```python
from build123d import *

# Parameters (mm, degrees)
BOSS_EXTRUDE1_DEPTH = 10
SKETCH1_5_OUTSIDE_W = 85.55
SKETCH1_5_OUTSIDE_H = 68.8
CUT_EXTRUDE2_DEPTH  = 10
SKETCH5_R           = 2.25
CUT_EXTRUDE3_DEPTH  = 10


with BuildPart() as part:
    # Sketch1 → Boss-Extrude1 (new body)
    with BuildSketch(Plane(origin=(0, 0, 0), x_dir=(0, 0, -1), z_dir=(1, 0, 0))):
        with BuildLine():
            Line((7.980196803, 33.697050156), (-4.769859567, -10.767680589))
            ThreePointArc((-4.769859567, -10.767680589), (-4.949582903, -11.029179666), (-5.250490415, -11.129861911))
            Line((-5.250490415, -11.129861911), (-12.87371339, -11.129861911))
            ThreePointArc((-12.87371339, -11.129861911), (-13.227266781, -11.276308521), (-13.37371339, -11.629861911))
            Line((-13.37371339, -11.629861911), (-13.37371339, -14.129861911))
            Line((-13.37371339, -14.129861911), (25.12628661, -14.129861911))
            Line((25.12628661, -14.129861911), (25.12628661, -11.629861911))
            ThreePointArc((25.12628661, -11.629861911), (24.979840001, -11.276308521), (24.62628661, -11.129861911))
            Line((24.62628661, -11.129861911), (17.12628661, -11.129861911))
            ThreePointArc((17.12628661, -11.129861911), (16.772733219, -10.983415302), (16.62628661, -10.629861911))
            Line((16.62628661, -10.629861911), (16.62628661, 27.870138089))
            ThreePointArc((16.62628661, 27.870138089), (17.504966266, 29.991458432), (19.62628661, 30.870138089))
            Line((19.62628661, 30.870138089), (53.37628661, 30.870138089))
            Line((53.37628661, 30.870138089), (53.37628661, 31.870138089))
            ThreePointArc((53.37628661, 31.870138089), (43.37628661, 32.880343233), (33.780368668, 35.870138089))
            Line((33.780368668, 35.870138089), (10.863981891, 35.870138089))
            ThreePointArc((10.863981891, 35.870138089), (9.058536822, 35.266044619), (7.980196803, 33.697050156))
        make_face()
    extrude(amount=BOSS_EXTRUDE1_DEPTH)

    # Sketch1_5 outside → Cut-Extrude2 (cut)
    # profile 1 of 2: a face of its own
    with BuildSketch(Plane(origin=(0, 0, 0), x_dir=(0, 0, -1), z_dir=(1, 0, 0))):
        with Locations((20.001, 10.87)):
            Rectangle(SKETCH1_5_OUTSIDE_W, SKETCH1_5_OUTSIDE_H)
        with BuildLine():
            Line((7.980196803, 33.697050156), (-4.769859567, -10.767680589))
            ThreePointArc((-4.769859567, -10.767680589), (-4.949582903, -11.029179666), (-5.250490415, -11.129861911))
            Line((-5.250490415, -11.129861911), (-12.87371339, -11.129861911))
            ThreePointArc((-12.87371339, -11.129861911), (-13.227266781, -11.276308521), (-13.37371339, -11.629861911))
            Line((-13.37371339, -11.629861911), (-13.37371339, -14.129861911))
            Line((-13.37371339, -14.129861911), (25.12628661, -14.129861911))
            Line((25.12628661, -14.129861911), (25.12628661, -11.629861911))
            ThreePointArc((25.12628661, -11.629861911), (24.979840001, -11.276308521), (24.62628661, -11.129861911))
            Line((24.62628661, -11.129861911), (17.12628661, -11.129861911))
            ThreePointArc((17.12628661, -11.129861911), (16.772733219, -10.983415302), (16.62628661, -10.629861911))
            Line((16.62628661, -10.629861911), (16.62628661, 27.870138089))
            ThreePointArc((16.62628661, 27.870138089), (17.504966266, 29.991458432), (19.62628661, 30.870138089))
            Line((19.62628661, 30.870138089), (53.37628661, 30.870138089))
            Line((53.37628661, 30.870138089), (53.37628661, 31.870138089))
            ThreePointArc((53.37628661, 31.870138089), (43.37628661, 32.880343233), (33.780368668, 35.870138089))
            Line((33.780368668, 35.870138089), (10.863981891, 35.870138089))
            ThreePointArc((10.863981891, 35.870138089), (9.058536822, 35.266044619), (7.980196803, 33.697050156))
        make_face(mode=Mode.SUBTRACT)
    # profile 2 of 2: a face of its own
    with BuildSketch(Plane(origin=(0, 0, 0), x_dir=(0, 0, -1), z_dir=(1, 0, 0))):
        with BuildLine():
            Line((0.9913062, -11.129861911), (11.12628661, -11.129861911))
            ThreePointArc((11.12628661, -11.129861911), (11.479840001, -10.983415302), (11.62628661, -10.629861911))
            Line((11.62628661, -10.629861911), (11.62628661, 24.715015158))
            ThreePointArc((11.62628661, 24.715015158), (11.195873161, 25.210149192), (10.645655762, 24.852833836))
            Line((10.645655762, 24.852833836), (0.510675352, -10.492043234))
            ThreePointArc((0.510675352, -10.492043234), (0.591988445, -10.930769423), (0.9913062, -11.129861911))
        make_face()
    extrude(amount=CUT_EXTRUDE2_DEPTH, mode=Mode.SUBTRACT)

    # Sketch5 → Cut-Extrude3 (cut)
    with BuildSketch(Plane.XZ.offset(14.129861911)):
        with Locations(Location((5, 9.12371339, 0), (0, 0, 270))):
            Circle(SKETCH5_R)
        with Locations(Location((5, -20.87628661, 0), (0, 0, 270))):
            Circle(SKETCH5_R)
    extrude(amount=-CUT_EXTRUDE3_DEPTH, mode=Mode.SUBTRACT)


solid = part.part
```
Check sheet for the modelled part. Datum: model origin and axes. Units: mm. A direction names the side the tool comes from. Round coordinates to 2 decimals unless told otherwise and drop trailing zeros. Loops run counter-clockwise (first coordinate to the right, second up) from the corner with the lowest first, then second, coordinate; pieces in that order, holes last. Notation, with made-up numbers: (-25, 6.5) -> (19, 6.5) arc R27 ccw to (19, 37.5) -> close; hole circle Ø8 at (44, 64.25). An arc over 180 degrees is marked (long way). Answer in a Markdown table with one row per item.
Q1. Set-up check for faces 1 (the face through (4.93, 7.43, -5.65)), 2 (the face through (2.7, -11.13, -21.8)), 3 (the face through (2.7, -11.13, 8.2)): record each of +Z, -Z, +X, -X, +Y, -Y from which the full face is reachable in a straight line by a thin tool's end or side.
Data:
| item | result |
|---|---|
| face 1 | +X, -X |
| face 2 | -Z, +X, -X |
| face 3 | +Z, +X, -X, +Y |
Q2. Sectioned sample at C-C on z = -2. Enter the section's corners in (x, y), then the cut area to 3 significant figures.
Data:
| item | result |
|---|---|
| outline | (0, -14.13) -> (10, -14.13) -> (10, -11.13) -> (0, -11.13) -> close; (0, -5.3) -> (10, -5.3) -> (10, 12.84) -> (0, 12.84) -> close |
| area | 211 mm^2 |
Q3. Thickness scan on L1, parallel to Z at x = 3.25, y = -9.5; L2, parallel to Z at x = 2.25, y = 2; L3, parallel to Y at x = 5.25, z = -17. Record the ranges inside material, lowest first.
Data:
| item | result |
|---|---|
| L1 | z = -16.63 to -11.63, -0.8 to 4.41 |
| L2 | z = -16.63 to -11.63, -4.09 to 1.11 |
| L3 | y = -14.13 to -11.11, 29.32 to 35.87 |
Q4. Sectioned sample at B-B on x = 2. Enter the section's corners in (y, z).
Data:
| item | result |
|---|---|
| outline | (-14.13, -25.13) -> (-11.63, -25.13) arc R0.5 ccw to (-11.13, -24.63) -> (-11.13, -17.13) arc R0.5 cw to (-10.63, -16.63) -> (27.87, -16.63) arc R3 cw to (30.87, -19.63) -> (30.87, -53.38) -> (31.87, -53.38) arc R50 cw to (35.87, -33.78) -> (35.87, -10.86) arc R3 ccw to (33.7, -7.98) -> (-10.77, 4.77) arc R0.5 cw to (-11.13, 5.25) -> (-11.13, 12.87) arc R0.5 ccw to (-11.63, 13.37) -> (-14.13, 13.37) -> close; hole (-11.13, -11.13) arc R0.5 ccw to (-10.63, -11.63) -> (24.72, -11.63) arc R0.5 ccw to (24.85, -10.65) -> (-10.49, -0.51) arc R0.5 ccw to (-11.13, -0.99) -> close |
Q5. Release check for a two-part mould opening along Z. For faces 4 (the face through (5, -13, 13.374)), 5 (the face through (5.68, -12.65, 6.98)), 6 (the face through (5, 8, -16.626)), 7 (the face through (0, 13, -12)) record: released by +Z, released by -Z, zero draft, split by the parting line, or undercut.
Data:
| item | result |
|---|---|
| face 4 | released by +Z |
| face 5 | undercut |
| face 6 | released by -Z |
| face 7 | zero draft |
Q6. Sectioned sample at A-A on x = 5. Give the number of separate pieces and of enclosed holes in the cut face, then the cut area to 3 significant figures.
Data:
| item | result |
|---|---|
| separate pieces | 3 |
| enclosed holes | 1 |
| area | 693 mm^2 |
Q7. Sectioned sample at D-D on y = -6. Enter the section's corners in (x, z).
Data:
| item | result |
|---|---|
| outline | (0, -16.63) -> (10, -16.63) -> (10, -11.63) -> (0, -11.63) -> close; (0, -1.8) -> (10, -1.8) -> (10, 3.4) -> (0, 3.4) -> close |
Q8. Go/stop test with flat-tipped pins: P1, Ø2, axis at x = 4.5, y = -13, coming from the -Z side; P2, Ø2, axis at x = 6.5, z = -31, coming from the -Y side; P3, Ø2, axis at x = 4.5, y = 27, coming from the +Z side; P4, Ø1, axis at y = -0.5, z = 2.5, coming from the +X side. Record where each tip stops, or that it passes through.
Data:
| item | result |
|---|---|
| P1 | stops at z = -25.13 |
| P2 | stops at y = 30.87 |
| P3 | stops at z = -5.77 |
| P4 | passes through |
